Part model, mm, in its own coordinate system. A direction names the side the tool comes from. Coordinates: 2 decimals unless noted, no trailing zeros. Order: outer loops, then holes, each group sorted by start corner. A loop starts at its lowest first (then second) coordinate and runs counter-clockwise, first axis right, second up. Notation, with made-up numbers: (21.25, 71) - (48.25, 71) arc R27 cw to (48.25, 106) - close; hole circle Ø11 at (4.5, 40). An arc over 180 degrees is marked (long way). Use a Markdown table: item, result. Add a question column.
1) Tool access for faces 4 (the face through (-21, 0, 60)), 5 (the face through (10, 72, 110)), 6 (the face through (-19.062, 96.166, 103.297)): list every direction of +Z, -Z, +X, -X, +Y, -Y with a clear straight run to the whole face (end or side of a thin tool).
2) Saw through at C-C on z = 17. List the corners of the cut face in (x, y), then the cut area to 3 significant figures.
3) Drop flat-ended pins along their axis: P1, Ø15, axis at y = -1.5, z = 101, coming from the -X side; P2, Ø4.5, axis at x = -14.5, z = 108, coming from the -Y side; P3, Ø4, axis at x = -30.5, y = -17.5, coming from the -Z side; P4, Ø13.5, axis at y = 80, z = 110, coming from the +X side. Give the stop position or say it passes through.
4) Saw through at A-A on x = -14. List the corners of the cut face in (y, z), then the cut area to 3 significant figures.
5) Saw through at D-D on z = 87. List the corners of the cut face in (x, y).
6) Saw through at B-B on y = 0. Count the separate pieces of the cut face and the enclosed holes in it, then the cut area to 4 significant figures.
7) Wall check: L1, parallel to Z at x = -28, y = 0; L2, parallel to X at y = 4, z = -25.5; L3, parallel to Z at x = 33.5, y = 0. Give the ranges that are in metal, low to high. Write a range as [from, to].
8) Two-plate mould, pull along X, no slides. Class faces 1 (the face through (-20, -27, 3)), 2 (the face through (0, -25, 56)), 3 (the face through (-20, 55, 110)): +X half, -X half, draft (parallel to the pull), parting line (faces both ways), or undercut.
Autodesk Fusion 360 part; units mm, degrees
sketch "Sketch1" plane through (0, 0, 0) normal (0, 1, 0) x (1, 0, 0)
  circle A0 centre (0, 0) radius 12.5
  circle A1 centre (0, 0) radius 25
  circle A2 centre (0, 110) radius 25
  circle A3 centre (0, 110) radius 40
  circle A4 centre (-80, 0) radius 7.5
  circle A5 centre (-80, 0) radius 17.5
  dimension "d1" = 25
  dimension "d2" = 50
  dimension "d3" = 50
  dimension "d4" = 80
  dimension "d5" = 15
  dimension "d6" = 35
  dimension "d7" = 110
  dimension "d8" = 80
sketch "Sketch2" plane through (0, 0, 0) normal (1, 0, 0) x (0, 1, 0)
  circle A0 centre (0, 0) radius 25
  circle A1 centre (0, 0) radius 40
  circle A2 centre (0, 110) radius 12.5
  circle A3 centre (0, 110) radius 25
  circle A4 centre (80, 110) radius 7.5
  circle A5 centre (80, 110) radius 17.5
  dimension "d19" = 50
  dimension "d20" = 80
  dimension "d21" = 25
  dimension "d22" = 50
  dimension "d23" = 15
  dimension "d24" = 35
  dimension "d25" = 110
  dimension "d26" = 80
  dimension "d27" = 110
extrude "Extrude6" add sketch "Sketch2" against normal blind 20 from surface at -20 contours A1 makes body 1
extrude "Extrude7" add sketch "Sketch2" against normal blind 15 from surface at -10 separate body contours A5 makes body 2
extrude "Extrude8" add sketch "Sketch2" along normal mid plane 60 separate body contours A3 makes body 3
mirror "Mirror1" about plane through (0, 0, 0) normal (1, 0, 0) of bodies 2 1 makes body 4 at (20, 97.413, 108.2576) makes body 5 at (33.3333, 39.9503, -1.9938)
sketch "Sketch3" plane through (0, 0, 0) normal (0, 1, 0) x (1, 0, 0)
  line L0 (40, 0) -> (40, -40)
  line L1 (40, 40) -> (40, 0)
  line L2 (20, 0) -> (20, 40)
  line L3 (20, -40) -> (20, 0)
  line L4 (40, 40) -> (20, 40)
  line L5 (40, -40) -> (20, -40)
  line L6 (-40, 0) -> (-40, -40)
  line L7 (-40, 40) -> (-40, 0)
  line L8 (-20, 0) -> (-20, 40)
  line L9 (-20, -40) -> (-20, 0)
  line L10 (-20, 40) -> (-40, 40)
  line L11 (-20, -40) -> (-40, -40)
  line L12 (-30, -110) -> (-30, -135)
  line L13 (-30, -85) -> (-30, -110)
  line L14 (30, -110) -> (30, -85)
  line L15 (30, -135) -> (30, -110)
  line L16 (-30, -135) -> (30, -135)
  line L17 (-30, -85) -> (30, -85)
  line L18 (-20, 0) -> (-35, 0)
  line L19 (-35, 0) -> (-35, -45)
  line L20 (-35, -45) -> (-20, -45)
  line L21 (-20, -45) -> (-20, 0)
  line L22 (20, 0) -> (35, 0)
  line L23 (35, 0) -> (35, -45)
  line L24 (35, -45) -> (20, -45)
  line L25 (20, -45) -> (20, 0)
  line L26 (35, -45) -> (-35, -45)
  line L27 (-35, -45) -> (-35, -60)
  line L28 (-35, -60) -> (35, -60)
  line L29 (35, -60) -> (35, -45)
  line L30 (7.5, -45) -> (-7.5, -45)
  line L31 (-7.5, -45) -> (-7.5, -110)
  line L32 (-7.5, -110) -> (7.5, -110)
  line L33 (7.5, -110) -> (7.5, -45)
  dimension "d38" = 15
  dimension "d39" = 45
  dimension "d40" = 15
  dimension "d41" = 45
  dimension "d42" = 15
  dimension "d43" = 15
  dimension "d44" = 65
  dimension "d45" = 27.5
extrude "Extrude9" add sketch "Sketch3" along normal mid plane 50 separate body contours L5 L23 L24 L25 L26 | L3 L5 L22 L23 L25 | L24 L26 L28 L29 L33 | L26 L28 L30 L31 L33 | L17 L28 L31 L33 | L20 L26 L27 L28 L31 | L17 L31 L32 L33 | L11 L19 L20 L21 L26 | L9 L11 L18 L19 L21 makes body 6
extrude "Extrude10" cut sketch "Sketch2" along normal through all and the other way through all contours A0 | A2 bodies 6
ref_plane "WorkPlane1" through (-17.5, 80, 110) normal (0, 0, -1) x (-1, 0, 0)
sketch "Sketch4" plane through (0, 0, 110) normal (0, 0, -1) x (-1, 0, 0)
  line L0 (-25, 62.5) -> (-25, 97.5)
  line L1 (-10, 97.5) -> (-10, 62.5)
  line L2 (-25, 62.5) -> (-10, 62.5)
  line L3 (-25, 97.5) -> (-10, 97.5)
  line L4 (25, 62.5) -> (25, 97.5)
  line L5 (10, 97.5) -> (10, 62.5)
  line L6 (10, 62.5) -> (25, 62.5)
  line L7 (10, 97.5) -> (25, 97.5)
  line L8 (30, -25) -> (30, 25)
  line L9 (-30, 25) -> (-30, -25)
  line L10 (30, 25) -> (-30, 25)
  line L11 (30, -25) -> (-30, -25)
  line L12 (10, 80) -> (20, 80)
  line L13 (20, 80) -> (20, 55)
  line L14 (20, 55) -> (10, 55)
  line L15 (10, 55) -> (10, 80)
  line L16 (-10, 80) -> (-20, 80)
  line L17 (-20, 80) -> (-20, 55)
  line L18 (-20, 55) -> (-10, 55)
  line L19 (-10, 55) -> (-10, 80)
  line L20 (-20, 55) -> (20, 55)
  line L21 (20, 55) -> (20, 45)
  line L22 (20, 45) -> (-20, 45)
  line L23 (-20, 45) -> (-20, 55)
  line L24 (-5, 55) -> (5, 55)
  line L25 (5, 55) -> (5, 0)
  line L26 (5, 0) -> (-5, 0)
  line L27 (-5, 0) -> (-5, 55)
  dimension "d50" = 10
  dimension "d51" = 25
  dimension "d52" = 10
  dimension "d53" = 25
  dimension "d54" = 10
  dimension "d55" = 10
  dimension "d56" = 55
  dimension "d57" = 15
  dimension "d58" = 15
extrude "Extrude11" add sketch "Sketch4" along normal mid plane 35 separate body contours L1 L2 L16 L17 L19 | L2 L17 L18 L19 L20 | L18 L20 L22 L23 L27 | L20 L22 L24 L25 L27 | L10 L22 L25 L27 | L14 L20 L21 L22 L25 | L10 L25 L26 L27 | L6 L13 L14 L15 L20 | L5 L6 L12 L13 L15 makes body 7
extrude "Extrude12" cut sketch "Sketch2" along normal through all and the other way through all contours A2 | A4 bodies 7
combine "Combine1" operation add target body 3 tool bodies 6 7 2 5 1 4
Results are:
| question | item | result |
|---|---|---|
| 1 | face 4 | -X, +Y, -Y |
| 1 | face 5 | +Z, -Z, +Y |
| 1 | face 6 | -X |
| 2 | outline | (-40, -36.21) - (-20, -36.21) - (-20, -18.33) - (-40, -18.33) - close; (-40, 18.33) - (-20, 18.33) - (-20, 36.21) - (-40, 36.21) - close; (20, -36.21) - (40, -36.21) - (40, -18.33) - (20, -18.33) - close; (20, 18.33) - (40, 18.33) - (40, 36.21) - (20, 36.21) - close |
| 2 | area | 1,430 mm2 |
| 3 | P1 | x = -30 |
| 3 | P2 | y = -25 |
| 3 | P3 | z = -36.87 |
| 3 | P4 | through |
| 4 | outline | (-25, 45) - (25, 45) - (25, 60) - (-25, 60) - close; circle Ø50 at (0, 110); (45, 92.5) - (80, 92.5) arc R17.5 ccw to (80, 127.5) - (45, 127.5) - close; hole circle Ø25 at (0, 110); hole circle Ø15 at (80, 110) |
| 4 | area | 3,750 mm2 |
| 5 | outline | (-30, -9.8) - (-7.5, -9.8) - (-7.5, -25) - (7.5, -25) - (7.5, -9.8) - (30, -9.8) - (30, 9.8) - (7.5, 9.8) - (7.5, 25) - (-7.5, 25) - (-7.5, 9.8) - (-30, 9.8) - close |
| 6 | separate pieces | 4 |
| 6 | enclosed holes | 0 |
| 6 | area | 4,275 mm2 |
| 7 | L1 | [-40, -25], [25, 60], [85, 97.5], [122.5, 135] |
| 7 | L2 | [-40, -20], [20, 40] |
| 7 | L3 | [-40, -25], [25, 60] |
| 8 | face 1 | undercut |
| 8 | face 2 | draft |
| 8 | face 3 | -X half |
